The model under review builds one solid part; all positions refer to its coordinate system, in mm. Face numbers are marked on the shaded views. A direction names the side the tool comes from. Coordinates: 2 decimals unless noted, no trailing zeros. Write each loop counter-clockwise with the first axis right and the second up, starting at its lowest first coordinate (ties: lowest second). Pieces come first, ordered by that corner, then holes. Notation, with made-up numbers: (32, 76) - (57, 76) arc R22 ccw to (57, 89) - close; hole circle Ø6 at (54, 35.25). An arc over 180 degrees is marked (long way). Put each result on its own line as item: value. Start each with the question number.
Item 1: Consider section B-B on y = -315.5. Give the boundary of the cut face in (x, z), then the cut area to 3 significant figures.
Item 2: Machinability: for the marked faces 1 and 2, which of the approach directions +Z, -Z, +X, -X, +Y, -Y give a long, thin tool a straight path to every point of the face, cutting with its end or side? Answer none if there is none.
Item 3: For pin 1 (18.5 mm diameter, centred on x = 13.5, z = 51.5, fed in from -Y); pin 2 (6 mm diameter, centred on x = 9.5, y = -380, fed in from +Z), all flat-tipped, find the tip position at first contact; note any pin that passes through.
Item 4: Consider section C-C on z = 10. Give the boundary of the cut face in (x, y), then the cut area to 3 significant figures.
Item 5: Consider section A-A on x = 2.5. Give the boundary of the cut face in (y, z), then the cut area to 3 significant figures.
Item 6: To check wall thickness, follow L1, parallel to Z at x = 51, y = -300.5; L2, parallel to Y at x = 48, z = 39. State the ranges of each line that lie inside material, in increasing order. Write a range as [from, to].
```python
from build123d import *

# Parameters (mm, degrees)
SKETCH_1_W      = 180
SKETCH_1_H      = 1350
EXTRUDE_1_DEPTH = 10
SKETCH_2_W      = 180
SKETCH_2_H      = 675
EXTRUDE_2_DEPTH = 200
SCALE_1_SCALE   = 0.345


with BuildPart() as part:
    # 草图1 → 凸台-拉伸1 (new body)
    with BuildSketch(Plane.XY):
        with Locations((76.977478815, -652.957853403)):
            Rectangle(SKETCH_1_W, SKETCH_1_H)
    extrude(amount=EXTRUDE_1_DEPTH)

    # 草图2 → 凸台-拉伸2 (add)
    with BuildSketch(Plane.XY.offset(10)):
        with Locations((76.977478815, -315.457853403)):
            Rectangle(SKETCH_2_W, SKETCH_2_H)
    extrude(amount=EXTRUDE_2_DEPTH)


with BuildPart() as part_1:
    # 缩放比例1: scaled about (0, 0, 0)
    add(part.part.scale(SCALE_1_SCALE))


solid = part_1.part
```
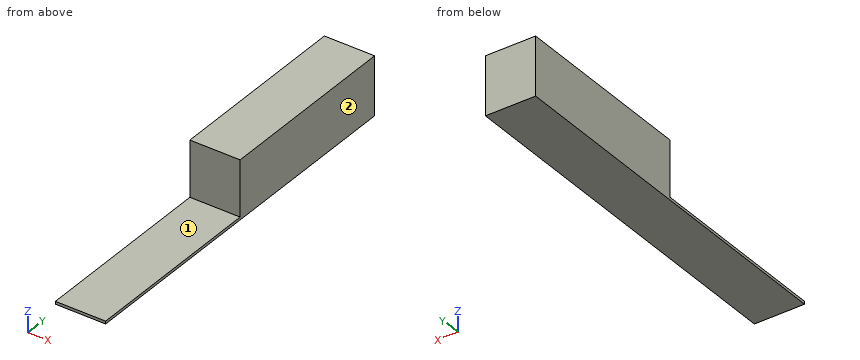
Report:
1. outline: (-4.49, 0) - (57.61, 0) - (57.61, 3.45) - (-4.49, 3.45) - close
1. area: 214 mm²
2. face 1: +Z, +X, -X, -Y
2. face 2: +Z, -Z, +X, +Y, -Y
3. pin 1: y = -225.27
3. pin 2: z = 3.45
4. outline: (-4.49, -225.27) - (57.61, -225.27) - (57.61, 7.6) - (-4.49, 7.6) - close
4. area: 14,500 mm²
5. outline: (-458.15, 0) - (7.6, 0) - (7.6, 72.45) - (-225.27, 72.45) - (-225.27, 3.45) - (-458.15, 3.45) - close
5. area: 17,700 mm²
6. L1: [0, 3.45]
6. L2: [-225.27, 7.6]
